Verification items for the finished model (mm, model axes). A direction names the side the tool comes from. Round coordinates to 2 decimals unless told otherwise and drop trailing zeros. Order: outer loops, then holes, each group sorted by start corner. A loop starts at its lowest first (then second) coordinate and runs counter-clockwise, first axis right, second up. Notation, with made-up numbers: (71, 37) -> (75, 37) arc R26 cw to (75, 52) -> close; hole circle Ø3 at (-28, 25). An arc over 180 degrees is marked (long way). Put each result on its own line as item: value.
```python
from build123d import *

# Parameters (mm, degrees)
SKETCH015_W   = 50
SKETCH015_H   = 40
SKETCH015_W_2 = 15
SKETCH015_H_2 = 15
PAD008_DEPTH  = 200


with BuildPart() as part:
    # Sketch015 → Pad008 (new body)
    with BuildSketch(Plane.YZ):
        with Locations((0, -0.005687)):
            Rectangle(SKETCH015_W, SKETCH015_H)
        with Locations((0, -6.005687)):
            Rectangle(SKETCH015_W_2, SKETCH015_H_2, mode=Mode.SUBTRACT)
    extrude(amount=PAD008_DEPTH)


with BuildPart() as part_1:
    # Body004 placement: moved
    add(part.part.moved(Location((28.722813, 0, 42.00053))))


solid = part_1.part
```
Item 1: Release check for a two-part mould opening along Y. For faces 3 (the face through (127, 25, 42)), 4 (the face through (127, 0, 43.495)), 5 (the face through (28.723, 0, 47)), 6 (the face through (127, 7.5, 36)) record: pulls with the +Y half, pulls with the -Y half, needs draft (parallel to the pull), parting line crosses it, or undercut.
Geometry check:
face 3: pulls with the +Y half
face 4: undercut
face 5: needs draft
face 6: undercut
Item 2: Material ranges on line 1 along Y through (x, z) = (122, 30); line 2 along Z through (x, y) = (126.5, 6), recorded low to high.
Geometry check:
line 1: -25 to -7.5, 7.5 to 25
line 2: 21.99 to 28.49, 43.49 to 61.99
Item 3: Sectioned sample at B-B, the plane x = 213. Record the boundary of the cut face in (y, z), then the cut area to 4 significant figures.
Geometry check:
outline: (-25, 21.99) -> (25, 21.99) -> (25, 61.99) -> (-25, 61.99) -> close; hole (-7.5, 28.49) -> (7.5, 28.49) -> (7.5, 43.49) -> (-7.5, 43.49) -> close
area: 1,775 mm2
Item 4: Tool access check on faces 1 (the face through (127, 0, 61.995)), 2 (the face through (127, 0, 28.495)). Record the directions out of +Z, -Z, +X, -X, +Y, -Y that give a thin tool (end or side, any length) a straight path to the whole face; none if there is none.
Geometry check:
face 1: +Z, +X, -X, +Y, -Y
face 2: +X, -X
Item 5: Sectioned sample at A-A, the plane y = 0. Record the boundary of the cut face in (x, z).
Geometry check:
outline: (28.72, 21.99) -> (228.72, 21.99) -> (228.72, 28.49) -> (28.72, 28.49) -> close; (28.72, 43.49) -> (228.72, 43.49) -> (228.72, 61.99) -> (28.72, 61.99) -> close
